Here's how the part is built. I have some questions about the finished solid (model axes, mm). A direction names the side the tool comes from. Round coordinates to 2 decimals unless told otherwise and drop trailing zeros. Write each loop counter-clockwise with the first axis right and the second up, starting at its lowest first coordinate (ties: lowest second). Pieces come first, ordered by that corner, then holes. Notation, with made-up numbers: (62, 12) - (119, 12) arc R9 ccw to (119, 19) - close; hole circle Ø11 at (26.5, 34). An arc over 180 degrees is marked (long way). Write item = value, one per line. Start each with the question number.
Item 1: Which directions (+Z, -Z, +X, -X, +Y, -Y) give clear straight access to the entire face, cutting with the end or side of a thin tool? Please do faces 1 (the face through (37, 1, -27)), 2 (the face through (45, 0, -21)).
Item 2: If I drill on line 1 along Z through (x, y) = (33.5, 1.1); line 2 along X through (y, z) = (2, -13.5); line 3 along X through (y, z) = (2, -11), over which ranges is the centre line in solid material (lowest first)? Write a range as [from, to].
Item 3: If we section it at B-B (z = -46): Please give me the cut outline in (x, y).
Item 4: Thinking about a two-plate mould opening in Z: for faces 3 (the face through (67, 1, -27)), 4 (the face through (45, 3, -21)), which applies, pulls with the +Z half, pulls with the -Z half, needs draft (parallel to the pull), parting line crosses it, or undercut?
Item 5: If we section it at C-C (y = 1.6): Give the number of separate pieces and of enclosed holes in the cut face, and give its area (3 significant figures).
Item 6: If we section it at A-A (x = 46): Please give me the cut outline in (y, z) (3 decimals), and give its area (3 significant figures).
```python
from build123d import *

# Parameters (mm, degrees)
SKETCH1_W           = 92
SKETCH1_H           = 53.85
SKETCH1_R           = 1
SKETCH1_R_2         = 1.6
SKETCH1_W_2         = 3
SKETCH1_H_2         = 10
BOSS_EXTRUDE1_DEPTH = 3


with BuildPart() as part:
    # Sketch1 → Boss-Extrude1 (new body)
    with BuildSketch(Plane(origin=(0, 0, 0), x_dir=(1, 0, 0), z_dir=(0, 1, 0))):
        with Locations((46, 26.925)):
            Rectangle(SKETCH1_W, SKETCH1_H)
        with Locations(Location((46, 26.925, 0), (0, 0, 270))):
            Circle(SKETCH1_R, mode=Mode.SUBTRACT)
        with Locations(Location((30, 46, 0), (0, 0, 270))):
            Circle(SKETCH1_R_2, mode=Mode.SUBTRACT)
        with Locations(Location((67, 41.5, 0), (0, 0, 270))):
            Circle(SKETCH1_R_2, mode=Mode.SUBTRACT)
        with Locations(Location((67, 13.5, 0), (0, 0, 270))):
            Circle(SKETCH1_R_2, mode=Mode.SUBTRACT)
        with Locations(Location((30, 9, 0), (0, 0, 270))):
            Circle(SKETCH1_R_2, mode=Mode.SUBTRACT)
        with Locations((4.5, 43.85)):
            Rectangle(SKETCH1_W_2, SKETCH1_H_2, mode=Mode.SUBTRACT)
        with Locations((4.5, 10)):
            Rectangle(SKETCH1_W_2, SKETCH1_H_2, mode=Mode.SUBTRACT)
        with Locations((87.5, 10)):
            Rectangle(SKETCH1_W_2, SKETCH1_H_2, mode=Mode.SUBTRACT)
        with Locations((87.5, 43.85)):
            Rectangle(SKETCH1_W_2, SKETCH1_H_2, mode=Mode.SUBTRACT)
        with BuildLine():
            ThreePointArc((40.82182341, 29.955921841), (40, 26.925), (40.82182341, 23.894078159))
            ThreePointArc((40.82182341, 23.894078159), (42.190006482, 23.536202368), (42.547882273, 24.904385439))
            ThreePointArc((42.547882273, 24.904385439), (42, 26.925), (42.547882273, 28.945614561))
            ThreePointArc((42.547882273, 28.945614561), (42.190006482, 30.313797632), (40.82182341, 29.955921841))
        make_face(mode=Mode.SUBTRACT)
        with BuildLine():
            ThreePointArc((36.506676252, 32.481690042), (35, 26.925), (36.506676252, 21.368309958))
            ThreePointArc((36.506676252, 21.368309958), (37.874859324, 21.010434167), (38.232735115, 22.378617239))
            ThreePointArc((38.232735115, 22.378617239), (37, 26.925), (38.232735115, 31.471382761))
            ThreePointArc((38.232735115, 31.471382761), (37.874859324, 32.839565833), (36.506676252, 32.481690042))
        make_face(mode=Mode.SUBTRACT)
        with BuildLine():
            ThreePointArc((32.191529094, 35.007458242), (30, 26.925), (32.191529094, 18.842541758))
            ThreePointArc((32.191529094, 18.842541758), (33.559712166, 18.484665966), (33.917587957, 19.852849038))
            ThreePointArc((33.917587957, 19.852849038), (32, 26.925), (33.917587957, 33.997150962))
            ThreePointArc((33.917587957, 33.997150962), (33.559712166, 35.365334034), (32.191529094, 35.007458242))
        make_face(mode=Mode.SUBTRACT)
        with BuildLine():
            ThreePointArc((27.876381936, 37.533226443), (25, 26.925), (27.876381936, 16.316773557))
            ThreePointArc((27.876381936, 16.316773557), (29.244565008, 15.958897766), (29.602440799, 17.327080837))
            ThreePointArc((29.602440799, 17.327080837), (27, 26.925), (29.602440799, 36.522919163))
            ThreePointArc((29.602440799, 36.522919163), (29.244565008, 37.891102234), (27.876381936, 37.533226443))
        make_face(mode=Mode.SUBTRACT)
        with BuildLine():
            ThreePointArc((51.08533044, 30.1092447), (52, 26.925), (51.08533044, 23.7407553))
            ThreePointArc((51.08533044, 23.7407553), (49.707067917, 23.423907676), (49.390220294, 24.8021702))
            ThreePointArc((49.390220294, 24.8021702), (50, 26.925), (49.390220294, 29.0478298))
            ThreePointArc((49.390220294, 29.0478298), (49.707067917, 30.426092324), (51.08533044, 30.1092447))
        make_face(mode=Mode.SUBTRACT)
        with BuildLine():
            ThreePointArc((55.323105808, 32.76278195), (57, 26.925), (55.323105808, 21.08721805))
            ThreePointArc((55.323105808, 21.08721805), (53.944843284, 20.770370426), (53.627995661, 22.14863295))
            ThreePointArc((53.627995661, 22.14863295), (55, 26.925), (53.627995661, 31.70136705))
            ThreePointArc((53.627995661, 31.70136705), (53.944843284, 33.079629574), (55.323105808, 32.76278195))
        make_face(mode=Mode.SUBTRACT)
        with BuildLine():
            ThreePointArc((59.560881175, 35.416319201), (62, 26.925), (59.560881175, 18.433680799))
            ThreePointArc((59.560881175, 18.433680799), (58.182618651, 18.116833176), (57.865771028, 19.495095699))
            ThreePointArc((57.865771028, 19.495095699), (60, 26.925), (57.865771028, 34.354904301))
            ThreePointArc((57.865771028, 34.354904301), (58.182618651, 35.733166824), (59.560881175, 35.416319201))
        make_face(mode=Mode.SUBTRACT)
        with BuildLine():
            ThreePointArc((63.798656542, 38.069856451), (67, 26.925), (63.798656542, 15.780143549))
            ThreePointArc((63.798656542, 15.780143549), (62.420394018, 15.463295926), (62.103546395, 16.841558449))
            ThreePointArc((62.103546395, 16.841558449), (65, 26.925), (62.103546395, 37.008441551))
            ThreePointArc((62.103546395, 37.008441551), (62.420394018, 38.386704074), (63.798656542, 38.069856451))
        make_face(mode=Mode.SUBTRACT)
    extrude(amount=BOSS_EXTRUDE1_DEPTH)


solid = part.part
```
Reply:
q1.face_1 = +Y, -Y
q1.face_2 = +Z, -Z, +X, -X, -Y
q2.line_1 = [-53.85, -35.4], [-33.23, -20.62], [-18.45, 0]
q2.line_2 = [0, 3], [6, 65.4], [68.6, 86], [89, 92]
q2.line_3 = [0, 3], [6, 86], [89, 92]
q3.outline = (0, 0) - (3, 0) - (3, 3) - (0, 3) - close; (6, 0) - (28.4, 0) - (28.4, 3) - (6, 3) - close; (31.6, 0) - (86, 0) - (86, 3) - (31.6, 3) - close; (89, 0) - (92, 0) - (92, 3) - (89, 3) - close
q4.face_3 = undercut
q4.face_4 = needs draft
q5.separate_pieces = 1
q5.enclosed_holes = 17
q5.area = 4,560 mm2
q6.outline = (0, -53.85) - (3, -53.85) - (3, -27.925) - (0, -27.925) - close; (0, -25.925) - (3, -25.925) - (3, 0) - (0, 0) - close
q6.area = 156 mm2
